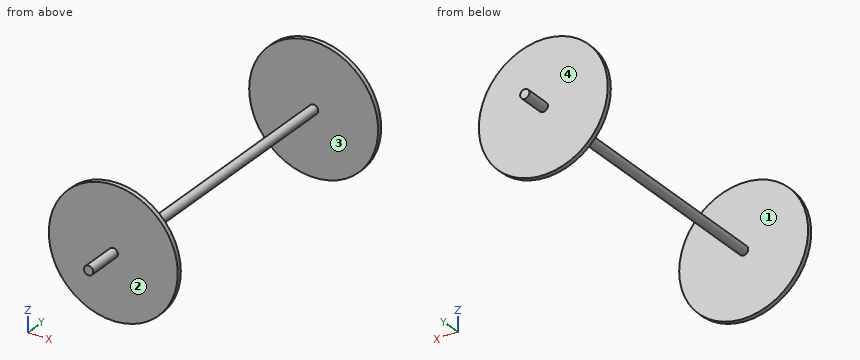
```python
from build123d import *

# Parameters (mm, degrees)
F0_R     = 3.175
F1_DEPTH = 203.2
F2_R     = 44.45
F3_DEPTH = 3.175
F4_R     = 44.45
F5_DEPTH = 3.175
F6_R     = 3.175
F7_DEPTH = 25.4
F8_R     = 3.175
F9_DEPTH = 19.05


with BuildPart() as f1:
    # F0 (on Front) → F1 (new body)
    with BuildSketch(Plane.XZ):
        Circle(F0_R)
    extrude(amount=F1_DEPTH)

    # F2 (on face) → F3 (join)
    with BuildSketch(Plane.XZ.offset(203.2)):
        Circle(F2_R)
    extrude(amount=F3_DEPTH)

    # F4 (on face) → F5 (join)
    with BuildSketch(Plane(origin=(0, 0, 0), x_dir=(-1, 0, 0), z_dir=(0, 1, 0))):
        Circle(F4_R)
    extrude(amount=F5_DEPTH)

    # F6 (on face) → F7 (join)
    with BuildSketch(Plane.XZ.offset(206.375)):
        Circle(F6_R)
    extrude(amount=F7_DEPTH)

    # F8 (on face) → F9 (join)
    with BuildSketch(Plane(origin=(0, 3.175, 0), x_dir=(-1, 0, 0), z_dir=(0, 1, 0))):
        Circle(F8_R)
    extrude(amount=F9_DEPTH)


solid = f1.part
```
Verification items for the finished model (mm, model axes). Face numbers are marked on the shaded views. Give positions to 0.01 mm unless a question says otherwise; leave off trailing zeros. Write each loop counter-clockwise with the first axis right and the second up, starting at its lowest first coordinate (ties: lowest second). Pieces come first, ordered by that corner, then holes. Notation, with made-up numbers: (41.25, 21.5) - (99.25, 21.5) arc R29 cw to (99.25, 41.5) - close; hole circle Ø3 at (84, 51). An arc over 180 degrees is marked (long way). Put each result on its own line as item: value.
Q1. Section check B-B on z = -36. Record the cut outline in (x, y) (3 decimals).
Result:
outline: (-26.073, -206.375) - (26.073, -206.375) - (26.073, -203.2) - (-26.073, -203.2) - close; (-26.073, 0) - (26.073, 0) - (26.073, 3.175) - (-26.073, 3.175) - close
Q2. Depth check by flat-ended pin: P1, Ø1, axis at x = -26, z = 6, coming from the -Y side (3 decimals); P2, Ø1, axis at x = -26, z = -30, coming from the +Y side (3 decimals); P3, Ø12, axis at y = -14, z = -10, coming from the +X side. Enter the tip coordinate at first touch or a pass-through.
Result:
P1: y = -206.375
P2: y = 3.175
P3: through
Q3. Mould release check, pull along Y, two halves, no side actions. Record for the marked faces 1, 2, 3 and 4: released by +Y, released by -Y, zero draft, split by the parting line, or undercut.
Result:
face 1: undercut
face 2: released by -Y
face 3: undercut
face 4: released by +Y
Q4. Section check D-D on x = 0. Record the cut outline in (y, z) (3 decimals), and give its area (3 significant figures).
Result:
outline: (-231.775, -3.175) - (-206.375, -3.175) - (-206.375, -44.45) - (-203.2, -44.45) - (-203.2, -3.175) - (0, -3.175) - (0, -44.45) - (3.175, -44.45) - (3.175, -3.175) - (22.225, -3.175) - (22.225, 3.175) - (3.175, 3.175) - (3.175, 44.45) - (0, 44.45) - (0, 3.175) - (-203.2, 3.175) - (-203.2, 44.45) - (-206.375, 44.45) - (-206.375, 3.175) - (-231.775, 3.175) - close
area: 2,140 mm2
Q5. Section check C-C on z = 0. Record the cut outline in (x, y) (3 decimals), and give its area (3 significant figures).
Result:
outline: (-44.45, -206.375) - (-3.175, -206.375) - (-3.175, -231.775) - (3.175, -231.775) - (3.175, -206.375) - (44.45, -206.375) - (44.45, -203.2) - (3.175, -203.2) - (3.175, 0) - (44.45, 0) - (44.45, 3.175) - (3.175, 3.175) - (3.175, 22.225) - (-3.175, 22.225) - (-3.175, 3.175) - (-44.45, 3.175) - (-44.45, 0) - (-3.175, 0) - (-3.175, -203.2) - (-44.45, -203.2) - close
area: 2,140 mm2
Q6. Scan lines: probe 1 along Y at (x, z) = (-1, -12.5) (3 decimals); probe 2 along Z at (x, y) = (0, -73.5) (3 decimals); probe 3 along Z at (x, y) = (1, -64). Record each from-to range of solid material in increasing order. Write a range as from..to.
Result:
probe 1: -206.375..-203.2, 0..3.175
probe 2: -3.175..3.175
probe 3: -3.01..3.01
Q7. Section check A-A on x = 24.5. Record the cut outline in (y, z) (3 decimals), and give its area (3 significant figures).
Result:
outline: (-206.375, -37.088) - (-203.2, -37.088) - (-203.2, 37.088) - (-206.375, 37.088) - close; (0, -37.088) - (3.175, -37.088) - (3.175, 37.088) - (0, 37.088) - close
area: 471 mm2
